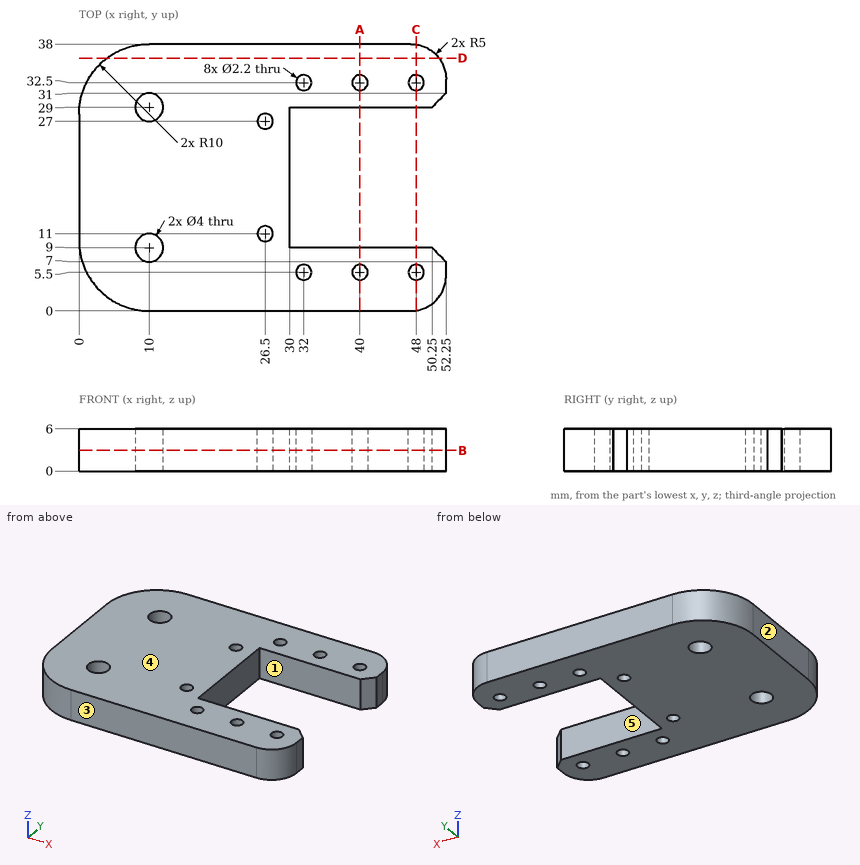
Verification items for this drawing (mm, ordinates from the low corner). A direction names the side the tool comes from. Give positions to 0.01 mm unless a question says otherwise; leave off trailing zeros. Loops run counter-clockwise (first coordinate to the right, second up) from the corner with the lowest first, then second, coordinate; pieces in that order, holes last. Notation, with made-up numbers: M 30.5,-17 L 81.5,-17 A24 ccw 81.5,22 Z; hole C -17.75,19.25 d6. An arc over 180 degrees is marked long. Answer as a JSON object with one key per item and string values. Group by question number.
Q1. Access from +Z, -Z, +X, -X, +Y, -Y to the whole of each face (thin tool, end or side, straight path). Record for the marked faces 4 and 5.
Q2. Go/stop test with flat-tipped pins: P1, Ø1, axis at x = 7, z = 0.5, coming from the -Y side; P2, Ø1.8, axis at x = 40, y = 5.5, coming from the -Z side; P3, Ø1.8, axis at y = 19.5, z = 2.5, coming from the +X side. Record where each tip stops, or that it passes through.
Q3. Cross-section at A-A on x = 40. Record the cut outline in (y, z).
Q4. Cross-section at B-B on z = 2.95. Give the number of separate pieces and of enclosed holes in the cut face, then the cut area to 3 significant figures.
Q5. Release check for a two-part mould opening along Y. For the marked faces 1, 2 and 3 record: released by +Y, released by -Y, zero draft, split by the parting line, or undercut.
Q6. Cross-section at C-C on x = 48. Record the cut outline in (y, z).
Q7. Cross-section at D-D on y = 36. Record the cut outline in (x, z).
Q8. Material ranges on line 1 along Y through (x, z) = (32, 1.95); line 2 along Y through (x, z) = (10, 2.55); line 3 along Y through (x, z) = (26.5, 2.6), recorded low to high. Write a range as [from, to].
Evaluation:
{
 "1": {"face 4": "+Z, +X, -X, +Y, -Y", "face 5": "+Z, -Z, +X"},
 "2": {"P1": "stops at y = 0.32", "P2": "passes through", "P3": "stops at x = 30"},
 "3": {"outline": "M 0,0 L 4.4,0 L 4.4,6 L 0,6 Z; M 6.6,0 L 9,0 L 9,6 L 6.6,6 Z; M 29,0 L 31.4,0 L 31.4,6 L 29,6 Z; M 33.6,0 L 38,0 L 38,6 L 33.6,6 Z"},
 "4": {"separate pieces": "1", "enclosed holes": "10", "area": "1,430 mm2"},
 "5": {"face 1": "undercut", "face 2": "zero draft", "face 3": "released by -Y"},
 "6": {"outline": "M 0.06,0 L 4.4,0 L 4.4,6 L 0.06,6 Z; M 6.6,0 L 9,0 L 9,6 L 6.6,6 Z; M 29,0 L 31.4,0 L 31.4,6 L 29,6 Z; M 33.6,0 L 37.94,0 L 37.94,6 L 33.6,6 Z"},
 "7": {"outline": "M 4,0 L 51.25,0 L 51.25,6 L 4,6 Z"},
 "8": {"line 1": "y = [0, 4.4], [6.6, 9], [29, 31.4], [33.6, 38]", "line 2": "y = [0, 7], [11, 27], [31, 38]", "line 3": "y = [0, 9.9], [12.1, 25.9], [28.1, 38]"}
}
